Geometry check sheet. Reference: the model listing, model coordinates, mm. A direction names the side the tool comes from. Give positions to 0.01 mm unless a question says otherwise; leave off trailing zeros. Answer in a Markdown table with one row per item. Add a question column.
```python
from build123d import *

# Parameters (mm, degrees)
F5_COUNT = 2
F5_ANGLE = 130
F7_R     = 1
F8_DEPTH = 1.901


with BuildPart() as f1:
    # F0 (on Front) → F1 (revolve)
    with BuildSketch(Plane.XZ):
        Polygon((8, 3.05), (8, 0), (16.65, 0), (18.107969, 1.457969), (17.215685, 1.697056), (19.195584, 3.676955), (19.434671, 2.784671), (20.5, 3.85), (20.5, 4.5), (18.2, 4.5), (18.2, 5.3), (17.5, 5.3), (17.5, 3), (16.35, 3), (16.35, 4.3), (15.6, 4.3), (15.6, 1.9), (11, 1.9), (11, 3.05), align=None)
    revolve(axis=Axis((0, 0, 2.65), (0, 0, 1)))


with BuildPart() as f4:
    # F4: sweep along a path in F3
    with BuildLine(Plane.XY.offset(3.05)) as f4_path:
        Line((0, -11), (0, 0))
    # F2 (on Front) → F4 (sweep)
    with BuildSketch(Plane.XZ):
        Polygon((-2.15, 3.05), (0, 0.9), (2.15, 3.05), align=None)
    sweep(path=f4_path.line)


with BuildPart() as f5_1:
    # F5: instance of F4
    add(f4.part.rotate(Axis((0, 0, 2.65), (0, 0, 1)), 1 * F5_ANGLE / (F5_COUNT - 1)))


with BuildPart() as f1_1:
    add(f1.part)

    # F6: cut F4, F5_1
    add(f4.part, mode=Mode.SUBTRACT)
    add(f5_1.part, mode=Mode.SUBTRACT)

    # F7 (on face) → F8 (cut, through all)
    with BuildSketch(Plane.XY.offset(1.9)):
        with Locations((0, -13.5)):
            Circle(F7_R)
        with Locations((8.649447, -10.365185)):
            Circle(F7_R)
    extrude(amount=-F8_DEPTH, mode=Mode.SUBTRACT)


solid = f1_1.part
```
1. Access from +Z, -Z, +X, -X, +Y, -Y to the whole of each face (thin tool, end or side, straight path). Record for faces 1 (the face through (7.91, -9.69, 0.96)), 2 (the face through (6.47, 6.81, 1.96)), 3 (the face through (-12.78, 11.72, 1.82)).
2. Release check for a two-part mould opening along X. For faces 4 (the face through (-15, 10, 5.3)), 5 (the face through (-4.444, -20.013, 4.18)), 6 (the face through (-13.887, -10.648, 4.134)) record: released by +X, released by -X, zero draft, split by the parting line, or undercut.
3. Material ranges on L1, parallel to Y at x = 0, z = 4.1; L2, parallel to Y at x = 0, z = 3.2; L3, parallel to Y at x = -13.5, z = 3.4, recorded low to high. Write a range as from..to.
4. Gauge pin test, flat ends, axial feed: pin 1 Ø2.5 at (x, y) = (8.65, -10.37) entering from -Z; pin 2 Ø9 at (x, y) = (-5, 0) entering from +Z; pin 3 Ø1 at (y, z) = (0, 3) entering from -X; pin 4 Ø1.5 at (x, z) = (2.5, 4.5) entering from -Y. Record the tip position at first contact, or that the pin passes through.
Response:
| question | item | result |
|---|---|---|
| 1 | face 1 | +Z, -Z |
| 1 | face 2 | +Z |
| 1 | face 3 | none |
| 2 | face 4 | zero draft |
| 2 | face 5 | split by the parting line |
| 2 | face 6 | undercut |
| 3 | L1 | y = -20.5..-17.5, -16.35..-15.6, 15.6..16.35, 17.5..20.5 |
| 3 | L2 | y = -19.85..-19.32, -18.72..-17.5, -16.35..-15.6, 15.6..16.35, 17.5..18.72, 19.32..19.85 |
| 3 | L3 | y = -14.82..-13.75, -13.25..-11.14, -9.22..-7.82, 7.82..9.22, 11.14..13.25, 13.75..14.82 |
| 4 | pin 1 | stops at z = 0 |
| 4 | pin 2 | stops at z = 3.05 |
| 4 | pin 3 | stops at x = -20.15 |
| 4 | pin 4 | stops at y = -20.43 |
